from build123d import *

# Parameters (mm, degrees)
BOSS_EXTRUDE1_DEPTH     = 385.705756272
SKETCH2_R               = 2.749999961
SKETCH2_R_2             = 14.2875
SKETCH2_R_3             = 2.75
CUT_EXTRUDE1_DEPTH      = 141.732
SKETCH14_R              = 3.302
CUT_EXTRUDE12_DEPTH     = 77.2
CUT_EXTRUDE13_DEPTH     = 101.6
SKETCH17_W              = 25.4
SKETCH17_H              = 25.4
CUT_EXTRUDE19_DEPTH     = 25.4
F_1_4_CLEARANCE_HOLE1_D = 6.7564
F_6_CLEARANCE_HOLE1_D   = 3.7973
CUT_EXTRUDE20_REACH     = 78.2
SKETCH25_W              = 25.4
SKETCH25_H              = 25.4
F_6_CLEARANCE_HOLE2_D   = 3.7973


with BuildPart() as part:
    # Sketch1 → Boss-Extrude1 (new body, symmetric)
    with BuildSketch(Plane(origin=(0, 0, 0), x_dir=(0, 0, -1), z_dir=(1, 0, 0))):
        Polygon((-38.1, 50.8), (38.1, 50.8), (38.1, -50.8), (34.925, -50.8), (34.925, 47.625), (-34.925, 47.625), (-34.925, -50.8), (-38.1, -50.8), align=None)
    extrude(amount=BOSS_EXTRUDE1_DEPTH, both=True)

    # Sketch2 → Cut-Extrude1 (cut)
    with BuildSketch(Plane.XY.offset(38.1)):
        with Locations((-333.475837626, -7.9375)):
            Circle(SKETCH2_R)
        with Locations((122.50039, -33.3375)):
            Circle(SKETCH2_R_2)
        with Locations((333.475837626, -7.9375)):
            Circle(SKETCH2_R)
        with Locations((334.902632555, -26.927596819)):
            Circle(SKETCH2_R_3)
        with Locations((-122.50039, -33.3375)):
            Circle(SKETCH2_R_2)
        with Locations((-334.902632555, -26.927596819)):
            Circle(SKETCH2_R_3)
    extrude(amount=-CUT_EXTRUDE1_DEPTH, mode=Mode.SUBTRACT)

    # Sketch14 → Cut-Extrude12 (cut, through all)
    with BuildSketch(Plane(origin=(0, 0, -38.1), x_dir=(-1, 0, 0), z_dir=(0, 0, -1))):
        with Locations((-160.60039, -35.123476108)):
            Circle(SKETCH14_R)
        with Locations((-160.61182, 41.076523035)):
            Circle(SKETCH14_R)
        with Locations((-84.41182, 41.076523892)):
            Circle(SKETCH14_R)
        with Locations((-84.41182, -35.123476108)):
            Circle(SKETCH14_R)
        with Locations((160.60039, -35.123476108)):
            Circle(SKETCH14_R)
        with Locations((84.41182, -35.123476108)):
            Circle(SKETCH14_R)
        with Locations((84.41182, 41.076523892)):
            Circle(SKETCH14_R)
        with Locations((160.61182, 41.076523035)):
            Circle(SKETCH14_R)
    extrude(amount=-CUT_EXTRUDE12_DEPTH, mode=Mode.SUBTRACT)

    # Sketch16 → Cut-Extrude13 (cut)
    with BuildSketch(Plane.XY.offset(38.1)):
        Polygon((-385.705756272, 25.4), (-341.71166576, -50.8), (-385.705756272, -50.8), align=None)
        Polygon((341.71166576, -50.8), (385.705756272, -50.8), (385.705756272, 25.4), align=None)
    extrude(amount=-CUT_EXTRUDE13_DEPTH, mode=Mode.SUBTRACT)

    # Sketch17 → Cut-Extrude19 (cut)
    with BuildSketch(Plane(origin=(0, 0, -38.1), x_dir=(-1, 0, 0), z_dir=(0, 0, -1))):
        with Locations((-12.7, 34.925)):
            Rectangle(SKETCH17_W, SKETCH17_H)
        with Locations((273.24, 34.925)):
            Rectangle(SKETCH17_W, SKETCH17_H)
    extrude(amount=-CUT_EXTRUDE19_DEPTH, mode=Mode.SUBTRACT)

    # 1/4 Clearance Hole1 (through all)
    with Locations(Plane(origin=(0, 0, -38.1), x_dir=(-1, 0, 0), z_dir=(0, 0, -1))):
        with Locations((-12.7, 34.925), (273.24, 34.925)):
            Hole(F_1_4_CLEARANCE_HOLE1_D / 2)

    # #6 Clearance Hole1 (through all)
    with Locations(Plane.XY.offset(38.1)):
        with Locations((-147.90039, -44.3), (-97.10039, -44.3), (97.10039, -44.3), (147.90039, -44.3), (-147.90039, 6.5), (-97.10039, 6.5), (97.10039, 6.5), (147.90039, 6.5)):
            Hole(F_6_CLEARANCE_HOLE1_D / 2)

    # Sketch25 → Cut-Extrude20 (cut, up to next)
    with BuildSketch(Plane.XY.offset(38.1), mode=Mode.PRIVATE) as cut_extrude20_sk1:
        with Locations((271.405756272, 34.925)):
            Rectangle(SKETCH25_W, SKETCH25_H)
    cut_extrude20_tool1 = extrude(cut_extrude20_sk1.sketch, amount=-CUT_EXTRUDE20_REACH, mode=Mode.PRIVATE) & part.part
    add(cut_extrude20_tool1.solids().sort_by_distance((271.405756, 34.925, 38.1))[0], mode=Mode.SUBTRACT)
    # Sketch25 → Cut-Extrude20 (cut, up to next)
    with BuildSketch(Plane.XY.offset(38.1), mode=Mode.PRIVATE) as cut_extrude20_sk2:
        with Locations((-271.405756272, 34.925)):
            Rectangle(SKETCH25_W, SKETCH25_H)
    cut_extrude20_tool2 = extrude(cut_extrude20_sk2.sketch, amount=-CUT_EXTRUDE20_REACH, mode=Mode.PRIVATE) & part.part
    add(cut_extrude20_tool2.solids().sort_by_distance((-271.405756, 34.925, 38.1))[0], mode=Mode.SUBTRACT)

    # #6 Clearance Hole2 (through all)
    with Locations(Plane.XY.offset(-34.925)):
        with Locations((-271.405756272, 34.925), (271.405756272, 34.925)):
            Hole(F_6_CLEARANCE_HOLE2_D / 2)


solid = part.part
Can you work these out from the model? Positions are in its coordinate system, mm. A direction names the side the tool comes from. Coordinates: 2 decimals unless noted, no trailing zeros. Write each loop counter-clockwise with the first axis right and the second up, starting at its lowest first coordinate (ties: lowest second). Pieces come first, ordered by that corner, then holes.
Q1. Please list where these lines run through material, in increasing order: L1, parallel to Z at x = -284, y = -14.5 (3 decimals); L2, parallel to Y at x = -157.5, z = 13.5 (3 decimals).
Results found:
L1: z = -38.1 to -34.925, 34.925 to 38.1
L2: y = 47.625 to 50.8
Q2. Which directions (+Z, -Z, +X, -X, +Y, -Y) give clear straight access to the entire face, cutting with the end or side of a thin tool? Please do faces 4 (the face through (5, -2, -34.925)), 5 (the face through (5, -1, 38.1)).
Results found:
face 4: +X, -X, -Y
face 5: +Z, +X, -X, +Y, -Y
Q3. For P1, Ø4.5, axis at x = -147.9, y = 6.5, coming from the +Z side; P2, Ø10, axis at y = -39.5, z = -30.5, coming from the +X side; P3, Ø3, axis at x = 152.5, z = 11.5, coming from the -Y side (3 decimals); P4, Ø3.5, axis at x = 334.9, y = -26.93, coming from the -Z side, each with a flat end and sliding along its axis, tell me the tip position at first contact or that it passes through.
Results found:
P1: stops at z = 38.1
P2: stops at x = 349.58
P3: stops at y = 47.625
P4: passes through
Q4. Imagine slicing it at A-A, the plane x = -38. List the corners of the cut face in (y, z) for me (3 decimals), plus the area to 3 significant figures.
Results found:
outline: (-50.8, -38.1) - (50.8, -38.1) - (50.8, 38.1) - (-50.8, 38.1) - (-50.8, 34.925) - (47.625, 34.925) - (47.625, -34.925) - (-50.8, -34.925) - close
area: 867 mm2
Q5. If we mould it in two halves opening along Y, with no side actions, what happens to faces 1 (the face through (111.16, -42.03, 36.53)), 2 (the face through (-364.017, -12.167, 36.535)), 3 (the face through (-385.706, 49, 0))? For each: +Y half, -Y half, draft (parallel to the pull), parting line (faces both ways), or undercut.
Results found:
face 1: undercut
face 2: -Y half
face 3: draft
Q6. Imagine slicing it at B-B, the plane z = -19. List the corners of the cut face in (x, y) for me (3 decimals), plus the area to 3 significant figures.
Results found:
outline: (-385.706, 47.625) - (385.706, 47.625) - (385.706, 50.8) - (-385.706, 50.8) - close
area: 2,450 mm2
